from build123d import *

# Parameters (mm, degrees)
SKETCH786_R             = 9.5
PAD342_DEPTH            = 31
SKETCH800_R             = 3.640093
SKETCH800_W             = 8.018949
SKETCH800_H             = 14.81283
SKETCH800_H_2           = 4.909163
POCKET216_DEPTH         = 8.316326
POCKET216_DEPTH_BACK    = 14.315221
SKETCH801_W             = 12.891265
SKETCH801_H             = 2.411679
SKETCH801_H_2           = 1.655072
SKETCH801_H_3           = 2.506252
SKETCH801_H_4           = 2.364388
POCKET217_DEPTH         = 14.211133
BODY063_PLACEMENT_ANGLE = 6


with BuildPart() as part:
    # Sketch786 → Pad342 (new body)
    with BuildSketch(Plane.XY.offset(62)):
        with BuildLine():
            Line((-6.48502, 14.210133), (14.314221, 11.983735))
            Line((14.314221, 11.983735), (13.827026, 7.082384))
            Line((13.827026, 7.082384), (14.121025, 4.779397))
            ThreePointArc((14.172916, 1.163416), (14.248889, 2.972869), (14.121025, 4.779397))
            Line((14.172916, 1.163416), (14.111788, 0.543408))
            ThreePointArc((13.818994, -0.764609), (14.005316, -0.119537), (14.111788, 0.543408))
            Line((13.818994, -0.764609), (12.909272, -3.318828))
            Line((12.122626, -4.979527), (12.909272, -3.318828))
            Line((10.986399, -7.012774), (12.122626, -4.979527))
            ThreePointArc((9.464654, -8.352981), (10.340262, -7.813155), (10.986399, -7.012774))
            Line((8.698858, -8.661427), (9.464654, -8.352981))
            ThreePointArc((5.823821, -9.218676), (7.288092, -9.078079), (8.698858, -8.661427))
            Line((2.72265, -9.218676), (5.823821, -9.218676))
            ThreePointArc((-0.561662, -8.908793), (1.073201, -9.141034), (2.72265, -9.218676))
            Line((-2.382517, -8.562102), (-0.561662, -8.908793))
            ThreePointArc((-4.482526, -7.588171), (-3.492747, -8.204996), (-2.382517, -8.562102))
            Line((-6.882625, -5.64591), (-4.482526, -7.588171))
            ThreePointArc((-7.614123, -4.427153), (-7.356079, -5.101176), (-6.882625, -5.64591))
            Line((-7.614123, -4.427153), (-8.095536, -1.933202))
            ThreePointArc((-8.235814, -0.549404), (-8.196714, -1.24445), (-8.095536, -1.933202))
            Line((-8.315326, 6.446385), (-8.235814, -0.549404))
            Line((-7.012325, 9.610864), (-8.315326, 6.446385))
            Line((-7.012325, 9.610864), (-6.48502, 14.210133))
        make_face()
        with Locations((2.566633, 2.779747)):
            Circle(SKETCH786_R, mode=Mode.SUBTRACT)
    extrude(amount=-PAD342_DEPTH)

    # Sketch800 → Pocket216 (cut, two sides)
    with BuildSketch(Plane.YZ) as pocket216_sk:
        with Locations((2.543955, 46.080971)):
            Circle(SKETCH800_R)
        with Locations((11.659285, 48.601678)):
            Rectangle(SKETCH800_W, SKETCH800_H)
        with Locations((11.659285, 32.332169)):
            Rectangle(SKETCH800_W, SKETCH800_H_2)
    extrude(amount=-POCKET216_DEPTH, mode=Mode.SUBTRACT)
    extrude(pocket216_sk.sketch, amount=POCKET216_DEPTH_BACK, mode=Mode.SUBTRACT)

    # Sketch801 → Pocket217 (cut, through all)
    with BuildSketch(Plane.XZ):
        with Locations((2.932228, 62.127093)):
            Rectangle(SKETCH801_W, SKETCH801_H)
        with Locations((2.932228, 30.93466)):
            Rectangle(SKETCH801_W, SKETCH801_H_2)
        with Locations((2.932228, 36.431635)):
            Rectangle(SKETCH801_W, SKETCH801_H_3)
        with Locations((2.932228, 53.693306)):
            Rectangle(SKETCH801_W, SKETCH801_H_4)
    extrude(amount=-POCKET217_DEPTH, mode=Mode.SUBTRACT)


with BuildPart() as part_1:
    # Body063 placement: moved
    add(part.part.moved(Location((1.045285, -9.945219, -20.5))).rotate(Axis((1.045285, -9.945219, -20.5), (0, 0, 1)), BODY063_PLACEMENT_ANGLE))


solid = part_1.part
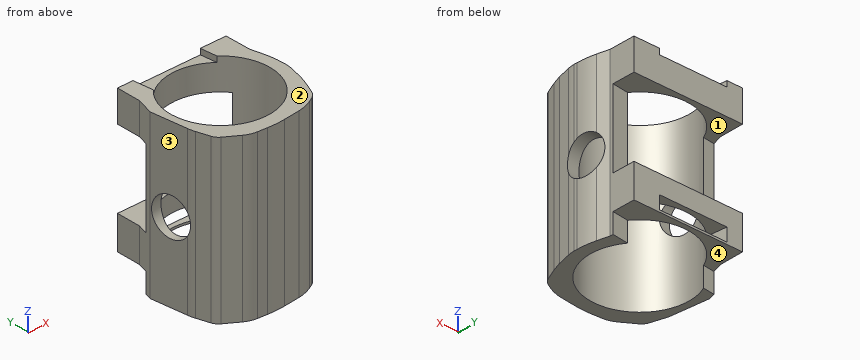
Can you work these out from the model? Positions are in its coordinate system, mm. Face numbers are marked on the shaded views. Give positions to 0.01 mm unless a question says otherwise; leave off trailing zeros. Write each loop counter-clockwise with the first axis right and the second up, starting at its lowest first coordinate (ties: lowest second). Pieces come first, ordered by that corner, then holes. Notation, with made-up numbers: M 57.5,30 L 99.5,30 A23 ccw 99.5,59 Z; hole C 48.5,55.5 d5. An arc over 180 degrees is marked long. Answer in a Markdown table with one row per item. Add a question column.
Item 1: Imagine slicing it at B-B, the plane x = -2. Write out the boundary of the cut face in (y, z).
Item 2: Imagine slicing it at D-D, the plane x = 8.25. Write out the boundary of the cut face in (y, z), plus the area to 3 significant figures.
Item 3: Imagine slicing it at C-C, the plane y = -14.75. Write out the boundary of the cut face in (x, z), plus the area to 3 significant figures.
Item 4: Imagine slicing it at A-A, the plane z = 13. Write out the boundary of the cut face in (x, y), plus the area to 3 significant figures.
Item 5: We'd pull the mould along Z, two halves only. Please class the marked faces 1, 2, 3 and 4: released by +Z, released by -Z, zero draft, split by the parting line, or undercut.
Item 6: For pin 1 Ø5.5 at (x, y) = (1, -1) entering from +Z; pin 2 Ø10 at (x, z) = (-5, 21) entering from -Y; pin 3 Ø4 at (x, y) = (3, 2) entering from +Z; pin 4 Ø2 at (y, z) = (-9, 23) entering from -X, each with a flat end and sliding along its axis, tell me the tip position at first contact or that it passes through.
Item 7: Please list where these lines run through material, in increasing order: L1, parallel to Z at x = 13.5, y = -0.25; L2, parallel to Y at x = 6.5, z = 20; L3, parallel to Z at x = 13.5, y = -6.5.
Evaluation:
| question | item | result |
|---|---|---|
| 1 | outline | M -18.3,10.5 L -14.79,10.5 L -14.79,41.5 L -18.3,41.5 Z; M 0.97,14.29 L 3.5,14.29 L 3.5,14.68 L 0.97,14.68 Z; M 0.97,17.18 L 3.5,17.18 L 3.5,20.7 L 0.97,20.7 Z; M 0.97,35.51 L 3.5,35.51 L 3.5,40.42 L 0.97,40.42 Z |
| 2 | outline | M -18.44,10.5 L -15.03,10.5 L -15.03,41.5 L -18.44,41.5 Z; M 1.2,14.29 L 3.48,14.29 L 3.48,14.68 L 1.2,14.68 Z; M 1.2,17.18 L 3.48,17.18 L 3.48,20.7 L 1.2,20.7 Z; M 1.2,35.51 L 3.48,35.51 L 3.48,40.42 L 1.2,40.42 Z |
| 2 | area | 126 mm² |
| 3 | outline | M -6.18,10.5 L -2.06,10.5 L -2.06,41.5 L -6.18,41.5 Z; M 8.68,10.5 L 13.14,10.5 L 13.14,41.5 L 8.68,41.5 Z |
| 3 | area | 266 mm² |
| 4 | outline | M -7.9,-4.4 L -7.09,-11.35 A7.77 ccw -6.8,-12.71 L -6.06,-15.14 A2.07 ccw -5.21,-16.28 L -2.62,-17.96 A4.75 ccw -0.43,-18.71 L 1.42,-18.86 A17.56 ccw 4.72,-18.83 L 7.8,-18.5 A7.7 ccw 10.6,-17.65 L 11.33,-17.26 A3.05 ccw 12.7,-15.77 L 13.62,-13.63 L 14.23,-11.9 L 14.87,-9.26 A5.51 ccw 15.02,-7.93 L 15.02,-7.31 A16.09 ccw 14.59,-3.72 L 14.06,-1.46 L 14.05,-0.89 L 10.91,-1.22 A9.5 cw long -5.31,-2.92 L -7.53,-3.15 Z |
| 4 | area | 110 mm² |
| 5 | face 1 | undercut |
| 5 | face 2 | released by +Z |
| 5 | face 3 | zero draft |
| 5 | face 4 | released by -Z |
| 6 | pin 1 | passes through |
| 6 | pin 2 | stops at y = -18.75 |
| 6 | pin 3 | stops at z = 40.42 |
| 6 | pin 4 | stops at x = -7.37 |
| 7 | L1 | z = 14.29 to 20.7, 35.51 to 41.5 |
| 7 | L2 | y = -18.64 to -15.86, 2.04 to 3.48 |
| 7 | L3 | z = 10.5 to 21.97, 29.2 to 41.5 |
